from build123d import *

# Parameters (mm, degrees)
SKETCH_1_W      = 42
SKETCH_1_H      = 20
SKETCH_1_R      = 2.5
EXTRUDE_1_DEPTH = 8
SKETCH_1_3_W    = 42
SKETCH_1_3_H    = 8
EXTRUDE_2_DEPTH = 30
SKETCH_2_W      = 42
SKETCH_2_H      = 71
SKETCH_2_R      = 1.5
SKETCH_2_R_2    = 11.5
EXTRUDE_3_DEPTH = 8


with BuildPart() as part:
    # 草图1 → 凸台-拉伸1 (new body)
    with BuildSketch(Plane.XY):
        with Locations((8.76, 8.6)):
            Rectangle(SKETCH_1_W, SKETCH_1_H)
        with Locations((-1.74, 8.6)):
            Circle(SKETCH_1_R, mode=Mode.SUBTRACT)
        with Locations((19.26, 8.6)):
            Circle(SKETCH_1_R, mode=Mode.SUBTRACT)
    extrude(amount=EXTRUDE_1_DEPTH)

    # 草图1<3> → 凸台-拉伸2 (add)
    with BuildSketch(Plane.XY):
        with Locations((8.76, -5.4)):
            Rectangle(SKETCH_1_3_W, SKETCH_1_3_H)
    extrude(amount=EXTRUDE_2_DEPTH)

    # 草图2 → 凸台-拉伸3 (add)
    with BuildSketch(Plane.XY.offset(30)):
        with Locations((8.76, 26.1)):
            Rectangle(SKETCH_2_W, SKETCH_2_H)
        with Locations((24.26, 56.1)):
            Circle(SKETCH_2_R, mode=Mode.SUBTRACT)
        with Locations((-6.74, 56.1)):
            Circle(SKETCH_2_R, mode=Mode.SUBTRACT)
        with Locations((-6.74, 25.1)):
            Circle(SKETCH_2_R, mode=Mode.SUBTRACT)
        with Locations((24.26, 25.1)):
            Circle(SKETCH_2_R, mode=Mode.SUBTRACT)
        with Locations((8.76, 40.6)):
            Circle(SKETCH_2_R_2, mode=Mode.SUBTRACT)
    extrude(amount=EXTRUDE_3_DEPTH)


solid = part.part
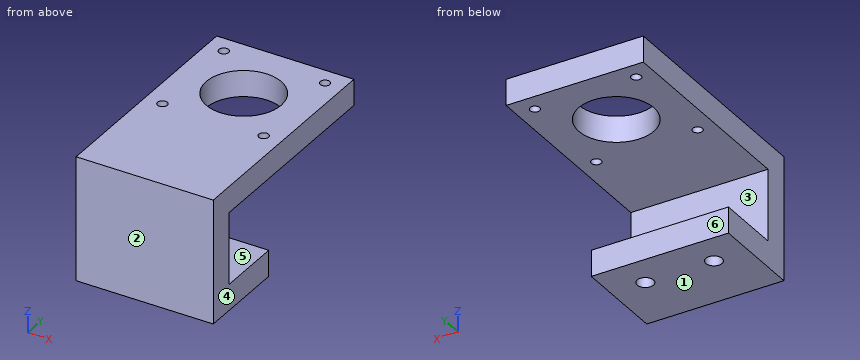
Here's how the part is built. I have some questions about the finished solid (model axes, mm). Face numbers are marked on the shaded views. A direction names the side the tool comes from. Give positions to 0.01 mm unless a question says otherwise; leave off trailing zeros. Loops run counter-clockwise (first coordinate to the right, second up) from the corner with the lowest first, then second, coordinate; pieces in that order, holes last. Notation, with made-up numbers: (16.5, -22.75) -> (47.5, -22.75) arc R36 ccw to (47.5, 15.25) -> close; hole circle Ø8 at (28, -26). An arc over 180 degrees is marked (long way). One line per item, written item: value.
Q1. On a 3-axis mill with a long thin cutter (end or side, diameter ignored), from which of +Z, -Z, +X, -X, +Y, -Y can I reach the whole of each face in a straight line? I mean the marked faces 4, 5 and 6. Say none if no direction works.
Answers follow:
face 4: +Z, -Z, +X, +Y, -Y
face 5: +X, -X, +Y
face 6: -Z, +X, -X, +Y
Q2. Suppose I cut it at D-D on x = 24.26. Please give me the cut outline in (y, z), then the cut area to 3 significant figures.
Answers follow:
outline: (-9.4, 0) -> (18.6, 0) -> (18.6, 8) -> (-1.4, 8) -> (-1.4, 30) -> (23.6, 30) -> (23.6, 38) -> (-9.4, 38) -> close; (26.6, 30) -> (54.6, 30) -> (54.6, 38) -> (26.6, 38) -> close; (57.6, 30) -> (61.6, 30) -> (61.6, 38) -> (57.6, 38) -> close
area: 920 mm^2
Q3. If I drill on line 1 along Z through (x, y) = (16.5, 6.5); line 2 along X through (y, z) = (8, 5); line 3 along Y through (x, z) = (13.5, 16.5), over which ranges is the centre line in solid material (lowest first)?
Answers follow:
line 1: 0 to 8, 30 to 38
line 2: -12.24 to -4.17, 0.69 to 16.83, 21.69 to 29.76
line 3: -9.4 to -1.4
Q4. Suppose I cut it at B-B on x = 8.76. Please give me the cut outline in (y, z).
Answers follow:
outline: (-9.4, 0) -> (18.6, 0) -> (18.6, 8) -> (-1.4, 8) -> (-1.4, 30) -> (29.1, 30) -> (29.1, 38) -> (-9.4, 38) -> close; (52.1, 30) -> (61.6, 30) -> (61.6, 38) -> (52.1, 38) -> close
Q5. I'm going to push flat-ended pins straight in: pin 1 Ø4 at (x, y) = (-6.74, 25.1) entering from -Z; pin 2 Ø6.5 at (x, z) = (12, 17.5) entering from +Y; pin 3 Ø4 at (x, z) = (17.5, 5.5) entering from +Y. Where does each tip first touch, or does it pass through?
Answers follow:
pin 1: z = 30
pin 2: y = -1.4
pin 3: y = 18.6
Q6. Suppose I cut it at C-C on y = 5. Please give me the cut outline in (x, z), then the cut area to 3 significant figures.
Answers follow:
outline: (-12.24, 0) -> (29.76, 0) -> (29.76, 8) -> (-12.24, 8) -> close; (-12.24, 30) -> (29.76, 30) -> (29.76, 38) -> (-12.24, 38) -> close
area: 672 mm^2
Q7. We'd pull the mould along Z, two halves only. Please class the marked faces 1, 2 and 3: pulls with the +Z half, pulls with the -Z half, needs draft (parallel to the pull), parting line crosses it, or undercut.
Answers follow:
face 1: pulls with the -Z half
face 2: needs draft
face 3: undercut
Q8. Suppose I cut it at A-A on y = 56.1. Please give me the cut outline in (x, z).
Answers follow:
outline: (-12.24, 30) -> (-8.24, 30) -> (-8.24, 38) -> (-12.24, 38) -> close; (-5.24, 30) -> (22.76, 30) -> (22.76, 38) -> (-5.24, 38) -> close; (25.76, 30) -> (29.76, 30) -> (29.76, 38) -> (25.76, 38) -> close
